Input: dimensioned drawing with shaded views. Units: mm. Origin: part minimum x, y, z. A direction names the side the tool comes from. Give positions to 0.01 mm unless a question says otherwise; leave off trailing zeros. Loops run counter-clockwise (first coordinate to the right, second up) from the corner with the lowest first, then second, coordinate; pieces in that order, holes last.
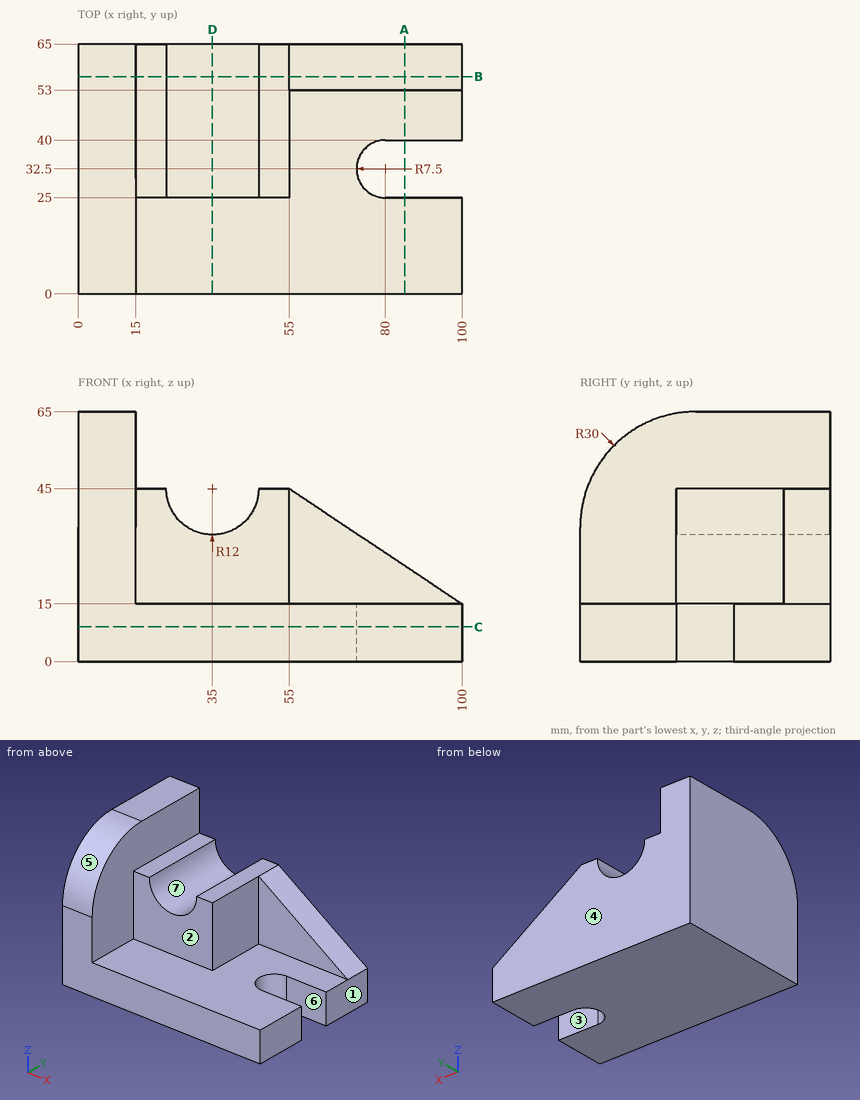
Item 1: Section query D-D on x = 35. Return loops of the section in (y, z).
Values follow:
outline: (0, 0) - (65, 0) - (65, 33) - (25, 33) - (25, 15) - (0, 15) - close
Item 2: Pin query (flat end, axial travel): pin 1 (12 mm diameter, centred on x = 58.5, z = 50.5, fed in from -Y); pin 2 (1.5 mm diameter, centred on x = 56.5, z = 20.5, fed in from -Y); pin 3 (24 mm diameter, centred on x = 36.5, z = 28, fed in from -Y); pin 4 (1.5 mm diameter, centred on x = 50, y = 21, fed in from +Z). Return the tip coordinate at first contact, or that it passes through.
Values follow:
pin 1: passes through
pin 2: stops at y = 53
pin 3: stops at y = 25
pin 4: stops at z = 15
Item 3: Ray query, probe 1 along X at (y, z) = (39, 48.5); probe 2 along Y at (x, z) = (53, 18); probe 3 along Z at (x, y) = (18.5, 61). Return the intervals inside material, ascending.
Values follow:
probe 1: x = 0 to 15
probe 2: y = 25 to 65
probe 3: z = 0 to 45
Item 4: Draft query along Y for the marked faces 4, 5, 6 and 7. Return one class per face: +Y half, -Y half, draft (parallel to the pull), parting line (faces both ways), or undercut.
Values follow:
face 4: +Y half
face 5: -Y half
face 6: undercut
face 7: draft
Item 5: Section query A-A on x = 85. Return loops of the section in (y, z).
Values follow:
outline: (0, 0) - (25, 0) - (25, 15) - (0, 15) - close; (40, 0) - (65, 0) - (65, 25) - (53, 25) - (53, 15) - (40, 15) - close
Item 6: Section query C-C on z = 9. Return loops of the section in (x, y), plus the area to 3 significant figures.
Values follow:
outline: (0, 0) - (100, 0) - (100, 25) - (80, 25) arc R7.5 cw to (80, 40) - (100, 40) - (100, 65) - (0, 65) - close
area: 6,110 mm2
Item 7: Set-up query: the marked faces 1, 2 and 3. Return all of +Z, -Z, +X, -X, +Y, -Y with unobstructed straight access to the full face (end or side cutting, diameter ignored); none if empty.
Values follow:
face 1: +Z, -Z, +X, +Y, -Y
face 2: +Z, +X, -Y
face 3: +Z, -Z, +X
Item 8: Section query B-B on y = 56.5. Return loops of the section in (x, z), plus the area to 3 significant figures.
Values follow:
outline: (0, 0) - (100, 0) - (100, 15) - (55, 45) - (47, 45) arc R12 cw to (23, 45) - (15, 45) - (15, 65) - (0, 65) - close
area: 3,900 mm2
